Input: part model. Units: mm. Frame: model coordinates. A direction names the side the tool comes from. Round coordinates to 2 decimals unless told otherwise and drop trailing zeros. Loops run counter-clockwise (first coordinate to the right, second up) from the corner with the lowest first, then second, coordinate; pieces in that order, holes last. Notation, with made-up numbers: M 45.5,38.5 L 63.5,38.5 A16 ccw 63.5,65.5 Z; hole C -27,-17 d9. An arc over 180 degrees is marked long. Put each result on its own line as item: value. Start each with the question number.
1) Line query: probe 1 along X at (y, z) = (22, 3.25); probe 2 along Y at (x, z) = (1.5, -8); probe 3 along X at (y, z) = (2, -5.5). Output: solid intervals per line, ascending.
2) Section B-B on z = 0. Output: boundary loops of the cut face in (x, y).
3) Draft query along Z for faces 1 (the face through (2, 5.08, 0)), 2 (the face through (-9.92, 4.204, 7.606)), 3 (the face through (15, 32.5, 0)), 4 (the face through (9.677, 3.011, -4.584)). Return one class per face: +Z half, -Z half, draft (parallel to the pull), parting line (faces both ways), or undercut.
4) Pin query (flat end, axial travel): pin 1 (4 mm diameter, centred on x = -5, z = -10, fed in from +Y); pin 2 (6.5 mm diameter, centred on x = -15.5, z = -0.5, fed in from -Y); pin 3 (2.5 mm diameter, centred on x = 1.5, z = 0, fed in from +Y); pin 4 (12.5 mm diameter, centred on x = 2.5, y = 25.5, fed in from +Z). Return the tip coordinate at first contact, or that it passes through.
5) Section D-D on y = 9.5. Output: boundary loops of the cut face in (x, z).
6) Section C-C on y = 27.5. Output: boundary loops of the cut face in (x, z).
7) Reachability of faces 5 (the face through (-12, 30, 0)), 6 (the face through (0, 7.5, 7)), 7 (the face through (-4.24, 0.29, -7.24)) from +Z, -Z, +X, -X, +Y, -Y: full face, straight path, thin tool, end or side. Return the list, or none.
8) Section A-A on y = 13. Output: boundary loops of the cut face in (x, z).
from build123d import *

# Parameters (mm, degrees)
SKETCH1_R           = 12.5
BOSS_EXTRUDE1_DEPTH = 7.5
SKETCH2_W           = 35
SKETCH2_H           = 8.580767914
BOSS_EXTRUDE2_DEPTH = 25
SKETCH3_W           = 25
SKETCH3_H           = 8.580767914
CUT_EXTRUDE1_DEPTH  = 20
SKETCH4_R           = 2.5
BOSS_EXTRUDE3_DEPTH = 3.75
SKETCH5_R           = 2.5
BOSS_EXTRUDE4_DEPTH = 3.75
FILLET2_R           = 2.5
FILLET3_R           = 2.5
CHAMFER1_SIZE       = 5
CHAMFER2_SIZE       = 5
CUT_EXTRUDE2_DEPTH  = 5.08
FILLET4_R           = 1


with BuildPart() as part:
    # Sketch1 → Boss-Extrude1 (new body)
    with BuildSketch(Plane(origin=(0, 0, 0), x_dir=(1, 0, 0), z_dir=(0, 1, 0))):
        Circle(SKETCH1_R)
    extrude(amount=BOSS_EXTRUDE1_DEPTH)

    # Sketch2 → Boss-Extrude2 (add)
    with BuildSketch(Plane(origin=(0, 7.5, 0), x_dir=(1, 0, 0), z_dir=(0, 1, 0))):
        Rectangle(SKETCH2_W, SKETCH2_H)
    extrude(amount=BOSS_EXTRUDE2_DEPTH)

    # Sketch3 → Cut-Extrude1 (cut)
    with BuildSketch(Plane(origin=(0, 32.5, 0), x_dir=(1, 0, 0), z_dir=(0, 1, 0))):
        Rectangle(SKETCH3_W, SKETCH3_H)
    extrude(amount=-CUT_EXTRUDE1_DEPTH, mode=Mode.SUBTRACT)

    # Sketch4 → Boss-Extrude3 (add)
    with BuildSketch(Plane(origin=(-12.5, 0, 0), x_dir=(0, 0, -1), z_dir=(1, 0, 0))):
        with Locations((0, 27.5)):
            Circle(SKETCH4_R)
    extrude(amount=BOSS_EXTRUDE3_DEPTH)

    # Sketch5 → Boss-Extrude4 (add)
    with BuildSketch(Plane.ZY.offset(-12.5)):
        with Locations((0, 27.5)):
            Circle(SKETCH5_R)
    extrude(amount=BOSS_EXTRUDE4_DEPTH)

    # Fillet2
    fillet2_edges = [part.edges().sort_by_distance(p)[0] for p in [
        (-8.75, 27.5, 2.5),
    ]]
    fillet(fillet2_edges, radius=FILLET2_R)

    # Fillet3
    fillet3_edges = [part.edges().sort_by_distance(p)[0] for p in [
        (8.75, 27.5, -2.5),
    ]]
    fillet(fillet3_edges, radius=FILLET3_R)

    # Chamfer1
    chamfer1_edges = [part.edges().sort_by_distance(p)[0] for p in [
        (-12.5, 12.5, 0),
    ]]
    chamfer(chamfer1_edges, length=CHAMFER1_SIZE)

    # Chamfer2
    chamfer2_edges = [part.edges().sort_by_distance(p)[0] for p in [
        (12.5, 12.5, 0),
    ]]
    chamfer(chamfer2_edges, length=CHAMFER2_SIZE)

    # Sketch6 → Cut-Extrude2 (cut)
    with BuildSketch(Plane.XZ):
        with BuildLine():
            Line((7.750974756, -4.654886545), (11.657827753, -4.510548978))
            ThreePointArc((11.657827753, -4.510548978), (12.287653293, -2.294248579), (12.5, 0))
            ThreePointArc((12.5, 0), (12.287653293, 2.294248579), (11.657827753, 4.510548978))
            Line((11.657827753, 4.510548978), (7.750974756, 4.510548978))
            Line((7.750974756, 4.510548978), (-0.186525244, 9.09326674))
            Line((-0.186525244, 9.09326674), (-8.124025244, 4.510548978))
            Line((-8.124025244, 4.510548978), (-8.124025244, -4.654886545))
            Line((-8.124025244, -4.654886545), (-0.186525244, -9.237604307))
            Line((-0.186525244, -9.237604307), (7.750974756, -4.654886545))
        make_face()
    extrude(amount=-CUT_EXTRUDE2_DEPTH, mode=Mode.SUBTRACT)

    # Fillet4
    fillet4_edges = [part.edges().sort_by_distance(p)[0] for p in [
        (-12.5, 0, 0),
        (9.704401254, 0, 4.510548978),
        (9.704401254, 0, -4.582717762),
        (3.782224756, 0, -6.946245426),
        (-4.155275244, 0, -6.946245426),
        (-8.124025244, 0, -0.072168784),
        (-4.155275244, 0, 6.801907859),
        (3.782224756, 0, 6.801907859),
    ]]
    fillet(fillet4_edges, radius=FILLET4_R)


solid = part.part
Geometry results:
1. probe 1: x = -17.5 to -12.5, 12.5 to 17.5
1. probe 2: y = 5.08 to 7.5
1. probe 3: x = -11.22 to -6.66, 6.29 to 11.22
2. outline: M -17.5,7.5 L -12.5,7.5 L -12.5,1 A1 ccw -11.5,0 L -9.12,0 A1 ccw -8.12,1 L -8.12,5.08 L 12.5,5.08 L 12.5,7.5 L 17.5,7.5 L 17.5,32.5 L 12.5,32.5 L 12.5,30 L 11.25,30 A2.5 ccw 11.25,25 L 12.5,25 L 12.5,17.5 L 7.5,12.5 L -7.5,12.5 L -12.5,17.5 L -12.5,25 L -11.25,25 A2.5 ccw -11.25,30 L -12.5,30 L -12.5,32.5 L -17.5,32.5 Z
3. face 1: undercut
3. face 2: parting line
3. face 3: draft
3. face 4: undercut
4. pin 1: stops at y = 7.5
4. pin 2: stops at y = 0.35
4. pin 3: stops at y = 12.5
4. pin 4: passes through
5. outline: M -17.5,-4.29 L 17.5,-4.29 L 17.5,4.29 L -17.5,4.29 Z
6. outline: M -17.5,-4.29 L -12.5,-4.29 L -12.5,-2.5 L -11.25,-2.5 A2.5 ccw -11.25,2.5 L -12.5,2.5 L -12.5,4.29 L -17.5,4.29 Z; M 11.25,-2.5 L 12.5,-2.5 L 12.5,-4.29 L 17.5,-4.29 L 17.5,4.29 L 12.5,4.29 L 12.5,2.5 L 11.25,2.5 A2.5 ccw Z
7. face 5: none
7. face 6: +Z, +X, -X, +Y
7. face 7: -Y
8. outline: M -17.5,-4.29 L -8,-4.29 L -8,4.29 L -17.5,4.29 Z; M 8,-4.29 L 17.5,-4.29 L 17.5,4.29 L 8,4.29 Z
